Read the model definition and answer for the solid it produces. Units are mm, in the model's axes. Face numbers are marked on the shaded views. A direction names the side the tool comes from. Coordinates: 2 decimals unless noted, no trailing zeros. Order: outer loops, then holes, each group sorted by start corner. A loop starts at its lowest first (then second) coordinate and runs counter-clockwise, first axis right, second up. Notation, with made-up numbers: (82.5, 17.5) -> (102.5, 17.5) arc R24 cw to (102.5, 44.5) -> close; hole circle Ø8 at (65, -21). An arc over 180 degrees is marked (long way). Answer as a JSON object with one key per item and string values. Group by question number.
1) Given pin 1 (3 mm diameter, centred on y = 2, z = -201.5, fed in from -X); pin 2 (3 mm diameter, centred on y = 2, z = -200, fed in from +X); pin 3 (6 mm diameter, centred on x = 75.5, z = -143, fed in from +Y), each flat-ended and moving along its own axis, determine where each tip first touches the part or whether it passes through.
2) Section A-A on z = -76 is taken. Determine the outline of the cut face in (x, y).
3) Consider L1, parallel to Z at x = 66.5, y = 0.9; L2, parallel to X at y = 3.3, z = -5; L3, parallel to X at y = 28, z = -92.5. Determine where each line is inside the solid, lowest interval first.
4) A tool of negligible diameter and unlimited length cuts with its end or side. For the marked faces 4, 5 and 6, from which of +Z, -Z, +X, -X, +Y, -Y can it reach the whole face along a straight path? Write none if from no direction.
5) Section C-C on y = 17 is taken. Determine the outline of the cut face in (x, z).
6) Determine the mould class of the marked faces 1, 2 and 3 for opening direction Z: released by +Z, released by -Z, zero draft, split by the parting line, or undercut.
7) Section B-B on x = 142 is taken. Determine the outline of the cut face in (y, z).
8) Section D-D on x = 74 is taken. Determine the outline of the cut face in (y, z).
from build123d import *

# Parameters (mm, degrees)
BOSS_EXTRUDE1_DEPTH = 4
BOSS_EXTRUDE2_DEPTH = 30
SKETCH3_W           = 218.358496247
SKETCH3_H           = 47.347449782
CUT_EXTRUDE1_DEPTH  = 317.987381452
BOSS_EXTRUDE3_START = -30
BOSS_EXTRUDE3_DEPTH = 30
BOSS_EXTRUDE4_START = -30
BOSS_EXTRUDE4_DEPTH = 30
CUT_EXTRUDE2_REACH  = 303.911
SKETCH6_R           = 2.5
SKETCH7_R           = 8
CUT_EXTRUDE3_DEPTH  = 29
BOSS_EXTRUDE5_START = -30
BOSS_EXTRUDE5_DEPTH = 30
SKETCH9_R           = 2.5
CUT_EXTRUDE4_DEPTH  = 302.911399089
SKETCH10_R          = 10
CUT_EXTRUDE5_DEPTH  = 29
SKETCH11_W          = 40
SKETCH11_H          = 17
CUT_EXTRUDE6_DEPTH  = 32
SKETCH14_R          = 1.3
CUT_EXTRUDE9_DEPTH  = 10
SKETCH12_R          = 1
CUT_EXTRUDE10_DEPTH = 302.487135546
SKETCH16_W          = 35
SKETCH16_H          = 20
SKETCH16_W_2        = 20
SKETCH16_H_2        = 25
SKETCH16_W_3        = 30
SKETCH16_W_4        = 15
CUT_EXTRUDE11_DEPTH = 302.487135546


# Read off the part's stored shape, not the designer's step: Boss-Extrude3, Boss-Extrude4, Boss-Extrude5
with BuildPart() as part:
    # Sketch1 → Boss-Extrude1 (new body)
    with BuildSketch(Plane(origin=(0, 0, 0), x_dir=(1, 0, 0), z_dir=(0, 1, 0))):
        with BuildLine():
            ThreePointArc((210, 130), (105, 235), (0, 130))
            Line((0, 130), (210, 130))
        make_face()
        with BuildLine():
            Line((210, 130), (0, 130))
            ThreePointArc((0, 130), (105, 25), (210, 130))
        make_face()
        with BuildLine():
            Line((0, 130), (0, 0))
            Line((0, 0), (210, 0))
            Line((210, 0), (210, 130))
            ThreePointArc((210, 130), (105, 25), (0, 130))
        make_face()
    extrude(amount=BOSS_EXTRUDE1_DEPTH)

    # Sketch2 → Boss-Extrude2 (add)
    with BuildSketch(Plane(origin=(0, 4, 0), x_dir=(1, 0, 0), z_dir=(0, 1, 0))):
        with BuildLine():
            Line((210, 0), (210, 130))
            ThreePointArc((210, 130), (105, 235), (0, 130))
            Line((0, 130), (0, 0))
            Line((0, 0), (210, 0))
        make_face()
        with BuildLine():
            ThreePointArc((4, 130), (105, 231), (206, 130))
            Line((206, 130), (206, 4))
            Line((206, 4), (4, 4))
            Line((4, 4), (4, 130))
        make_face(mode=Mode.SUBTRACT)
    extrude(amount=BOSS_EXTRUDE2_DEPTH)

    # Sketch3 → Cut-Extrude1 (cut, through all)
    with BuildSketch(Plane(origin=(0, 34, 0), x_dir=(1, 0, 0), z_dir=(0, 1, 0))):
        with Locations((109.179248124, 237.903724891)):
            Rectangle(SKETCH3_W, SKETCH3_H)
    extrude(amount=-CUT_EXTRUDE1_DEPTH, mode=Mode.SUBTRACT)

    # Boss-Extrude3 outline → Boss-Extrude3 (add)
    with BuildSketch(Plane(origin=(0, 34, 0), x_dir=(1, 0, 0), z_dir=(0, 1, 0)).offset(BOSS_EXTRUDE3_START)):
        with BuildLine():
            Line((160.734254279, 214.23), (49.265745721, 214.23))
            ThreePointArc((49.265745721, 214.23), (45.760745723, 211.802877411), (42.361297108, 209.23))
            Line((42.361297108, 209.23), (167.638702892, 209.23))
            ThreePointArc((167.638702892, 209.23), (164.239254277, 211.802877411), (160.734254279, 214.23))
        make_face()
    extrude(amount=BOSS_EXTRUDE3_DEPTH)

    # Boss-Extrude4 outline → Boss-Extrude4 (add)
    with BuildSketch(Plane(origin=(0, 34, 0), x_dir=(1, 0, 0), z_dir=(0, 1, 0)).offset(BOSS_EXTRUDE4_START)):
        with BuildLine():
            ThreePointArc((42.361297108, 209.23), (38.626128036, 206.128241281), (35.044335216, 202.850565986))
            ThreePointArc((35.044335216, 202.850565986), (46.447220251, 201.380271613), (54.847774812, 209.23))
            Line((54.847774812, 209.23), (42.361297108, 209.23))
        make_face()
        with BuildLine():
            Line((167.638702892, 209.23), (155.152225188, 209.23))
            ThreePointArc((155.152225188, 209.23), (163.552779749, 201.380271613), (174.955664785, 202.850565987))
            ThreePointArc((174.955664785, 202.850565987), (171.373871964, 206.128241281), (167.638702892, 209.23))
        make_face()
    extrude(amount=BOSS_EXTRUDE4_DEPTH)

    # Sketch6 → Cut-Extrude2 (cut, up to next)
    with BuildSketch(Plane(origin=(0, 34, 0), x_dir=(1, 0, 0), z_dir=(0, 1, 0)), mode=Mode.PRIVATE) as cut_extrude2_sk1:
        with Locations(Location((43.986828471, 209.23, 0), (0, 0, 270))):
            Circle(SKETCH6_R)
    cut_extrude2_tool1 = extrude(cut_extrude2_sk1.sketch, amount=-CUT_EXTRUDE2_REACH, mode=Mode.PRIVATE) & part.part
    # Sketch6 → Cut-Extrude2 (cut, up to next)
    with BuildSketch(Plane(origin=(0, 34, 0), x_dir=(1, 0, 0), z_dir=(0, 1, 0)), mode=Mode.PRIVATE) as cut_extrude2_sk2:
        with Locations(Location((166.013171529, 209.23, 0), (0, 0, 270))):
            Circle(SKETCH6_R)
    cut_extrude2_tool2 = extrude(cut_extrude2_sk2.sketch, amount=-CUT_EXTRUDE2_REACH, mode=Mode.PRIVATE) & part.part
    add(cut_extrude2_tool1.solids().sort_by_distance((43.986828, 34, -209.23))[0], mode=Mode.SUBTRACT)
    add(cut_extrude2_tool2.solids().sort_by_distance((166.013172, 34, -209.23))[0], mode=Mode.SUBTRACT)

    # Sketch7 → Cut-Extrude3 (cut)
    with BuildSketch(Plane(origin=(0, 34, 0), x_dir=(1, 0, 0), z_dir=(0, 1, 0))):
        with Locations((42.307838608, 214.23)):
            Circle(SKETCH7_R)
        with Locations((167.692161392, 214.23)):
            Circle(SKETCH7_R)
    extrude(amount=-CUT_EXTRUDE3_DEPTH, mode=Mode.SUBTRACT)

    # Boss-Extrude5 outline → Boss-Extrude5 (add)
    with BuildSketch(Plane(origin=(0, 34, 0), x_dir=(1, 0, 0), z_dir=(0, 1, 0)).offset(BOSS_EXTRUDE5_START)):
        with BuildLine():
            Line((4, 4), (11.842719282, 4))
            ThreePointArc((11.842719282, 4), (8.838834765, 8.838834765), (4, 11.842719282))
            Line((4, 11.842719282), (4, 4))
        make_face()
        with BuildLine():
            ThreePointArc((206, 11.842719282), (201.161165235, 8.838834765), (198.157280718, 4))
            Line((198.157280718, 4), (206, 4))
            Line((206, 4), (206, 11.842719282))
        make_face()
    extrude(amount=BOSS_EXTRUDE5_DEPTH)

    # Sketch9 → Cut-Extrude4 (cut, through all)
    with BuildSketch(Plane(origin=(0, 34, 0), x_dir=(1, 0, 0), z_dir=(0, 1, 0))):
        with Locations(Location((5, 5, 0), (0, 0, 270))):
            Circle(SKETCH9_R)
        with Locations(Location((205, 5, 0), (0, 0, 270))):
            Circle(SKETCH9_R)
    extrude(amount=-CUT_EXTRUDE4_DEPTH, mode=Mode.SUBTRACT)

    # Sketch10 → Cut-Extrude5 (cut)
    with BuildSketch(Plane(origin=(0, 34, 0), x_dir=(1, 0, 0), z_dir=(0, 1, 0))):
        Circle(SKETCH10_R)
        with Locations((210, 0)):
            Circle(SKETCH10_R)
    extrude(amount=-CUT_EXTRUDE5_DEPTH, mode=Mode.SUBTRACT)

    # Sketch11 → Cut-Extrude6 (cut)
    with BuildSketch(Plane(origin=(0, 4, 0), x_dir=(1, 0, 0), z_dir=(0, 1, 0))):
        with Locations((105, 12.5)):
            Rectangle(SKETCH11_W, SKETCH11_H)
    extrude(amount=-CUT_EXTRUDE6_DEPTH, mode=Mode.SUBTRACT)

    # Sketch14 → Cut-Extrude9 (cut)
    with BuildSketch(Plane(origin=(0, 4, 0), x_dir=(1, 0, 0), z_dir=(0, 1, 0))):
        with Locations(Location((17.5, 86.643431732, 0), (0, 0, 270))):
            Circle(SKETCH14_R)
        with Locations(Location((66.5, 86.643431732, 0), (0, 0, 270))):
            Circle(SKETCH14_R)
        with Locations(Location((17.5, 28.643431732, 0), (0, 0, 270))):
            Circle(SKETCH14_R)
        with Locations(Location((66.5, 28.643431732, 0), (0, 0, 270))):
            Circle(SKETCH14_R)
    extrude(amount=-CUT_EXTRUDE9_DEPTH, mode=Mode.SUBTRACT)

    # Sketch12 → Cut-Extrude10 (cut, through all)
    with BuildSketch(Plane(origin=(0, 4, 0), x_dir=(1, 0, 0), z_dir=(0, 1, 0))):
        with Locations(Location((86.9, 170.810842956, 0), (0, 0, 270))):
            Circle(SKETCH12_R)
        with Locations(Location((167.35, 101.210842956, 0), (0, 0, 270))):
            Circle(SKETCH12_R)
        with Locations(Location((167.35, 170.910842956, 0), (0, 0, 270))):
            Circle(SKETCH12_R)
        with Locations(Location((87, 101.210842956, 0), (0, 0, 270))):
            Circle(SKETCH12_R)
    extrude(amount=-CUT_EXTRUDE10_DEPTH, mode=Mode.SUBTRACT)

    # Sketch16 → Cut-Extrude11 (cut, through all)
    with BuildSketch(Plane(origin=(0, 4, 0), x_dir=(1, 0, 0), z_dir=(0, 1, 0))):
        with Locations((105, 199.23)):
            Rectangle(SKETCH16_W, SKETCH16_H)
        with Locations((42, 141.73)):
            Rectangle(SKETCH16_W_2, SKETCH16_H_2)
        with Locations((151, 66.5)):
            Rectangle(SKETCH16_W_3, SKETCH16_H_2)
        with Locations((191, 136.73)):
            Rectangle(SKETCH16_W_4, SKETCH16_H_2)
    extrude(amount=-CUT_EXTRUDE11_DEPTH, mode=Mode.SUBTRACT)


solid = part.part
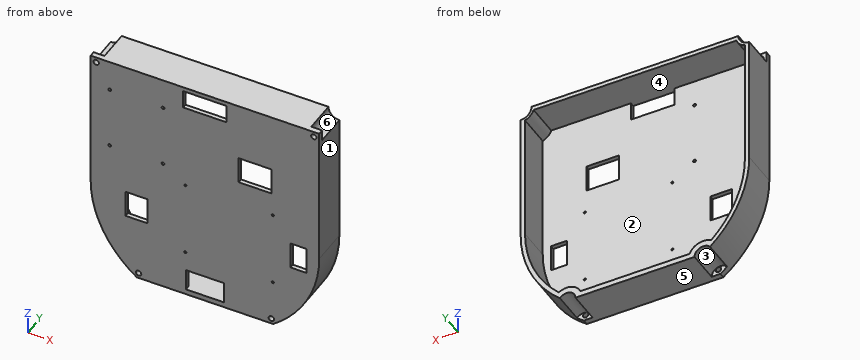
Worked answers:
{
 "1": {"pin 1": "stops at x = 26.74", "pin 2": "stops at x = 184.58", "pin 3": "stops at y = 4"},
 "2": {"outline": "(0, 0) -> (136, 0) -> (136, 4) -> (4, 4) -> (4, 34) -> (0, 34) -> close; (166, 0) -> (210, 0) -> (210, 34) -> (206, 34) -> (206, 4) -> (166, 4) -> close"},
 "3": {"L1": "z = -214.23 to -87.94, -85.34 to -29.94, -27.34 to 0", "L2": "x = 0 to 2.5, 7.5 to 85, 125 to 202.5, 207.5 to 210", "L3": "x = 0 to 4, 206 to 210"},
 "4": {"face 4": "+Y", "face 5": "-Z, +X, -X, +Y, -Y", "face 6": "+Z, +X, +Y"},
 "5": {"outline": "(0, -130) arc R105 ccw to (36.08, -209.21) arc R8 cw to (50.31, -214.23) -> (159.69, -214.23) arc R8 cw to (173.92, -209.21) arc R105 ccw to (210, -130) -> (210, -10) arc R10 cw to (200, 0) -> (10, 0) arc R10 cw to (0, -10) -> close; hole (4, -130) arc R101 ccw to (35.04, -202.85) arc R13.5 cw to (54.85, -209.23) -> (155.15, -209.23) arc R13.5 cw to (174.96, -202.85) arc R101 ccw to (206, -130) -> (206, -11.84) arc R12.5 cw to (198.16, -4) -> (11.84, -4) arc R12.5 cw to (4, -11.84) -> close"},
 "6": {"face 1": "zero draft", "face 2": "undercut", "face 3": "released by -Z"},
 "7": {"outline": "(0, -214.23) -> (34, -214.23) -> (34, -209.23) -> (4, -209.23) -> (4, -79) -> (0, -79) -> close; (0, -54) -> (4, -54) -> (4, -4) -> (34, -4) -> (34, 0) -> (0, 0) -> close"},
 "8": {"outline": "(0, -214.23) -> (34, -214.23) -> (34, -209.23) -> (4, -209.23) -> (4, -4) -> (34, -4) -> (34, 0) -> (0, 0) -> close"}
}
